Read the model definition and answer for the solid it produces. Units are mm, in the model's axes. A direction names the side the tool comes from. Coordinates: 2 decimals unless noted, no trailing zeros. Loops run counter-clockwise (first coordinate to the right, second up) from the corner with the lowest first, then second, coordinate; pieces in that order, holes last.
from build123d import *

# Parameters (mm, degrees)
F0_R     = 3.7313011015
F1_DEPTH = 5.08


# Not quite as in the source:
# - a feature names something its author has since deleted; it is built from what else it names


with BuildPart() as f1:
    # F0 (on Front) → F1 (new body)
    with BuildSketch(Plane.XZ):
        Polygon((-0.2968451337, 20.2413384518), (7.4894401646, 9.9239995871), (14.8768772094, 19.7128383483), (7.0905919112, 30.0301772131), (0, 39.4256766967), (-7.3874370448, 29.6368379354), (-14.8768772094, 19.7128383483), (-7.7862852982, 10.3173388647), align=None)
        Polygon((14.5800320757, 0.5285001035), (7.4894401646, 9.9239995871), (-0.2968451337, 20.2413384518), (-7.7862852982, 10.3173388647), (-15.1737223431, 0.5285001035), (-7.5532907703, -9.5690716936), (0, 0.4395341352), (7.2564456366, -9.175732416), align=None)
        Polygon((0, 39.4256766967), (7.0905919112, 30.0301772131), (14.5800320757, 39.9541768002), (7.4894401646, 49.3496762838), (-0.2968451337, 59.6670151485), (-7.7862852982, 49.7430155614), (-15.1737223431, 39.9541768002), (-7.3874370448, 29.6368379354), align=None)
        Polygon((14.8768772094, -19.2733042131), (7.2564456366, -9.175732416), (0, 0.4395341352), (-7.5532907703, -9.5690716936), (-14.8768772094, -19.2733042131), (-14.5568754898, -19.6973274863), (10.9024396727, -19.6973274863), (14.5568754898, -19.6973274863), align=None)
        Polygon((-0.2968451337, 59.6670151485), (7.4894401646, 49.3496762838), (15.3495463603, 59.7648326808), (0, 80.103988665), (-15.3495463602, 59.7648326808), (-7.7862852982, 49.7430155614), align=None)
        Polygon((6.4679318367, -25.5733413094), (10.9024396727, -19.6973274863), (-14.5568754898, -19.6973274863), (-13.9719483627, -20.4723943058), (-9.1415820241, -25.5733413094), (-1.0331695214, -19.9124130418), align=None)
        Polygon((18.6885435032, -25.5733413094), (10.9024396727, -19.6973274863), (6.4679318367, -25.5733413094), (-1.0331695214, -19.9124130418), (-9.1415820241, -25.5733413094), (-13.9719483627, -20.4723943058), (-14.7059016213, -19.6973274863), (-20.9110697187, -25.5733413094), (-26.4753893159, -19.6973274863), (-32.6805574134, -25.5733413094), (-38.2448770106, -19.6973274863), (-38.2448770106, -31.4493551324), (-8.4425376974, -31.4493551324), (5.4781014785, -31.4493551324), (5.6878598178, -31.4493551324), (39.2251229894, -31.4493551324), (39.2251229894, -19.6973274863), (30.4618320136, -25.5733413094), (22.9607306555, -19.9124130418), align=None)
        Polygon((5.4781014785, -31.7272986938), (5.6878598178, -31.4493551324), (5.4781014785, -31.4493551324), align=None)
        Polygon((5.4781014785, -58.5252254202), (5.4781014785, -31.7272986938), (5.4781014785, -31.4493551324), (-8.4425376974, -31.4493551324), (-8.4425376974, -58.5252254202), align=None)
        Polygon((19.711822737, -58.5252254202), (5.4781014785, -58.5252254202), (-8.4425376974, -58.5252254202), (-24.1670380346, -58.5252254202), (-2.355908975, -82.3924914002), align=None)
        with Locations((0, -67.5043612719)):
            Circle(F0_R, mode=Mode.SUBTRACT)
    extrude(amount=F1_DEPTH)


solid = f1.part
Q1. Flat-ended cylindrical pins translate along their axes: pin 1 Ø1 at (x, y) = (-24.5, -0.5) entering from +Z; pin 2 Ø2.5 at (x, y) = (29, -2) entering from -Z; pin 3 Ø1.5 at (y, z) = (-3.5, -46) entering from +X. Find the tip coordinate at first contact, or state that the pin passes through.
Findings below:
pin 1: stops at z = -21.26
pin 2: stops at z = -31.45
pin 3: stops at x = 5.48
Q2. Straight lines are drawn through the part: probe 1 along Z at (x, y) = (9.5, -4.4); probe 2 along X at (y, z) = (-2.2, -47.5); probe 3 along Z at (x, y) = (-22.5, -0.35). For each, find the intervals that lie inside material, in ascending order.
Findings below:
probe 1: z = -69.57 to -58.53, -31.45 to -12.15, -6.2 to 7.26, 12.59 to 26.84, 33.22 to 46.69, 52.01 to 67.52
probe 2: x = -8.44 to 5.48
probe 3: z = -60.35 to -58.53, -31.45 to -23.9
Q3. A cutting plane is placed at D-D (z = 63.5). Give the vertices of the cut face in (x, y).
Findings below:
outline: (-12.53, -5.08) - (12.53, -5.08) - (12.53, 0) - (-12.53, 0) - close
Q4. A cutting plane is placed at B-B (x = -18). Give the vertices of the cut face in (y, z), then the cut area to 3 significant figures.
Findings below:
outline: (-5.08, -65.27) - (0, -65.27) - (0, -58.53) - (-5.08, -58.53) - close; (-5.08, -31.45) - (0, -31.45) - (0, -22.82) - (-5.08, -22.82) - close
area: 78.1 mm2
Q5. A cutting plane is placed at C-C (z = -52.5). Give the vertices of the cut face in (x, y).
Findings below:
outline: (-8.44, -5.08) - (5.48, -5.08) - (5.48, 0) - (-8.44, 0) - close
Q6. Determine the mould class of faces 4 (the face through (39.225, -3, -26)), 5 (the face through (11.13, -2.5, 14.75)), 6 (the face through (20.855, -2.504, -22.703)) for opening direction Z: +Z half, -Z half, draft (parallel to the pull), parting line (faces both ways), or undercut.
Findings below:
face 4: draft
face 5: undercut
face 6: +Z half
Q7. A cutting plane is placed at A-A (x = 13). Give the vertices of the cut face in (y, z), then the cut area to 3 significant figures.
Findings below:
outline: (-5.08, -65.78) - (0, -65.78) - (0, -58.53) - (-5.08, -58.53) - close; (-5.08, -31.45) - (0, -31.45) - (0, -21.28) - (-5.08, -21.28) - close; (-5.08, -19.7) - (0, -19.7) - (0, -16.79) - (-5.08, -16.79) - close; (-5.08, -1.57) - (0, -1.57) - (0, 2.62) - (-5.08, 2.62) - close; (-5.08, 17.23) - (0, 17.23) - (0, 22.2) - (-5.08, 22.2) - close; (-5.08, 37.86) - (0, 37.86) - (0, 42.05) - (-5.08, 42.05) - close; (-5.08, 56.65) - (0, 56.65) - (0, 62.88) - (-5.08, 62.88) - close
area: 203 mm2
Q8. Which of the six approach directions +Z, -Z, +X, -X, +Y, -Y give full straight-line access (tool end or side, diameter ignored) to faces 1 (the face through (22, -3, -31.449)), 2 (the face through (-29.53, -2.5, -22.59)), 3 (the face through (-11.62, -2.5, 54.82))?
Findings below:
face 1: +X, +Y, -Y
face 2: +Z, +Y, -Y
face 3: -X, +Y, -Y
